from build123d import *

# Parameters (mm, degrees)
SKIZZE1_R                       = 0.75
AUFSATZ_LINEAR_AUSTRAGEN1_DEPTH = 1


with BuildPart() as part:
    # Skizze1 → Aufsatz-Linear austragen1 (new body)
    with BuildSketch(Plane.XY.offset(1)):
        with BuildLine():
            Line((-0.5, -8.084553173), (-0.5, -4.773887305))
            ThreePointArc((-0.5, -4.773887305), (0, 4.8), (0.5, -4.773887305))
            Line((0.5, -4.773887305), (0.5, -8.084553173))
            ThreePointArc((0.5, -8.084553173), (2.199840536, -7.79555653), (3.8, -7.153320907))
            Line((3.8, -7.153320907), (3.8, -4.385545471))
            ThreePointArc((3.8, -4.385545471), (0, 6.6), (-3.8, -4.385545471))
            Line((-3.8, -4.385545471), (-3.8, -7.153320907))
            ThreePointArc((-3.8, -7.153320907), (-2.199840536, -7.79555653), (-0.5, -8.084553173))
        make_face()
        with Locations(Location((1.98, -6.45, 0), (0, 0, 180))):
            Circle(SKIZZE1_R, mode=Mode.SUBTRACT)
        with Locations(Location((-1.98, -6.45, 0), (0, 0, 180))):
            Circle(SKIZZE1_R, mode=Mode.SUBTRACT)
    extrude(amount=-AUFSATZ_LINEAR_AUSTRAGEN1_DEPTH)


solid = part.part
CAD build for the part. Positions are in the model's coordinates, mm. A direction names the side the tool comes from. Round coordinates to 2 decimals unless told otherwise and drop trailing zeros. Loops run counter-clockwise (first coordinate to the right, second up) from the corner with the lowest first, then second, coordinate; pieces in that order, holes last.
(1) Cut at A-A (y = -5.5). Give the cut face in (x, z).
(2) Cut at C-C (x = -4.5). Give the cut face in (y, z), plus the area to 3 significant figures.
(3) Cut at B-B (z = 0.75). Give the cut face in (x, y), plus the area to 3 significant figures.
(4) Wall check: line 1 along X through (y, z) = (-6.45, 0.6); line 2 along Y through (x, z) = (-1.98, 0.8); line 3 along Y through (x, z) = (-1.5, 0.65). Give the ranges that are in metal, low to high.
(5) Two-plate mould, pull along X, no slides. Class faces 1 (the flat face through (3, -4, 1)), 2 (the flat face through (3.8, -5.8, 0.5)), 3 (the cylindrical face through (-1.817, -5.718, 0.507)): +X half, -X half, draft (parallel to the pull), parting line (faces both ways), or undercut.
(6) Drop a flat-ended pin along its axis: pin 1 (6 mm diameter, centred on x = 0, y = 0, fed in from -Z). Give the stop position or say it passes through.
(7) Cut at D-D (x = 1.98). Give the cut face in (y, z), plus the area to 3 significant figures.
(8) Which spindle directions (+Z, -Z, +X, -X, +Y, -Y) get a long thin tool onto all of the face, cutting with end or side? Do faces 4 (the flat face through (-3.8, -5.8, 0.5)), 5 (the cylindrical face through (2.143, -5.718, 0.507)), 6 (the flat face through (0.5, -6.4, 0.5)). Say none if no direction does.
Findings below:
1. outline: (-3.8, 0) - (-0.5, 0) - (-0.5, 1) - (-3.8, 1) - close; (0.5, 0) - (3.8, 0) - (3.8, 1) - (0.5, 1) - close
2. outline: (-3.74, 0) - (-1.67, 0) - (-1.67, 1) - (-3.74, 1) - close; (1.67, 0) - (4.64, 0) - (4.64, 1) - (1.67, 1) - close
2. area: 5.04 mm2
3. outline: (-3.8, -7.15) arc R8.1 ccw to (-0.5, -8.08) - (-0.5, -4.77) arc R4.8 cw (long way) to (0.5, -4.77) - (0.5, -8.08) arc R8.1 ccw to (3.8, -7.15) - (3.8, -4.39) arc R6.15 ccw (long way) to (-3.8, -4.39) - close; hole circle Ø1.5 at (-1.98, -6.45); hole circle Ø1.5 at (1.98, -6.45)
3. area: 58.7 mm2
4. line 1: x = -3.8 to -2.73, -1.23 to -0.5, 0.5 to 1.23, 2.73 to 3.8
4. line 2: y = -7.85 to -7.2, -5.7 to -4.37, 4.37 to 6.27
4. line 3: y = -7.96 to -7.03, -5.87 to -4.56, 4.56 to 6.41
5. face 1: draft
5. face 2: +X half
5. face 3: undercut
6. pin 1: passes through
7. outline: (-7.85, 0) - (-7.2, 0) - (-7.2, 1) - (-7.85, 1) - close; (-5.7, 0) - (-4.37, 0) - (-4.37, 1) - (-5.7, 1) - close; (4.37, 0) - (6.27, 0) - (6.27, 1) - (4.37, 1) - close
7. area: 3.88 mm2
8. face 4: +Z, -Z, -X, -Y
8. face 5: +Z, -Z
8. face 6: +Z, -Z, -Y
